```python
from build123d import *

# Parameters (mm, degrees)
F2_DEPTH = 25.4
F0_W     = 101.8392853439
F0_H     = 138.1853856146
F0_R     = 44.7370158625
F3_DEPTH = 25.4


with BuildPart() as f2:
    # F1 (on Right) → F2 (new body)
    with BuildSketch(Plane.YZ):
        with BuildLine():
            ThreePointArc((5.1872688346, 24.6414919816), (16.2456525152, 42.3484863922), (20.1080592166, 62.8645122051))
            ThreePointArc((20.1080592166, 62.8645122051), (-51.2286548469, 117.2754631001), (-84.8408640002, 34.0907424688))
            Line((-84.8408640002, 34.0907424688), (5.1872688346, 34.0907424688))
            Line((5.1872688346, 34.0907424688), (5.1872688346, 24.6414919816))
        make_face()
        with BuildLine():
            Line((5.1872688346, 34.0907424688), (-84.8408640002, 34.0907424688))
            ThreePointArc((-84.8408640002, 34.0907424688), (-42.2001575317, 6.7538301414), (5.1872688346, 24.6414919816))
            Line((5.1872688346, 24.6414919816), (5.1872688346, 34.0907424688))
        make_face()
        with BuildLine():
            ThreePointArc((5.1872688346, 24.6414919816), (-42.2001575317, 6.7538301414), (-84.8408640002, 34.0907424688))
            Line((-84.8408640002, 34.0907424688), (-98.5580086708, 34.0907424688))
            Line((-98.5580086708, 34.0907424688), (-98.5580086708, -30.617037788))
            Line((-98.5580086708, -30.617037788), (5.1872688346, -30.617037788))
            Line((5.1872688346, -30.617037788), (5.1872688346, 24.6414919816))
        make_face()
    extrude(amount=F2_DEPTH)

    # F0 (on Top) → F3 (join)
    with BuildSketch(Plane.XY):
        with Locations((-13.9607731253, -10.5434413999)):
            Rectangle(F0_W, F0_H)
        with Locations((-15.9663036466, 12.9214562476)):
            Circle(F0_R, mode=Mode.SUBTRACT)
    extrude(amount=F3_DEPTH)


solid = f2.part
```
Build history of the part. All positions in model axes, mm. A direction names the side the tool comes from. Give positions to 0.01 mm unless a question says otherwise; leave off trailing zeros. Loops run counter-clockwise (first coordinate to the right, second up) from the corner with the lowest first, then second, coordinate; pieces in that order, holes last.
Item 1: Slice it at A-A, the plane y = -23.5. List the corners of the cut face in (x, z), and give its area (3 significant figures).
Answers follow:
outline: (-64.88, 0) - (-41.94, 0) - (-41.94, 25.4) - (-64.88, 25.4) - close; (0, -30.62) - (25.4, -30.62) - (25.4, 0) - (36.96, 0) - (36.96, 25.4) - (25.4, 25.4) - (25.4, 117.81) - (0, 117.81) - close
area: 4,650 mm2
Item 2: Which spindle directions (+Z, -Z, +X, -X, +Y, -Y) get a long thin tool onto all of the face, cutting with end or side? Do faces 1 (the face through (31, -79.636, 13)), 2 (the face through (13, -98.558, 2)), 3 (the face through (-33, -79.636, 13)). Say none if no direction does.
Answers follow:
face 1: +Z, -Z, +X, -Y
face 2: +Z, -Z, +X, -X, -Y
face 3: +Z, -Z, -X, -Y
Item 3: Drill centre lines: line 1 (X direction, y = 5, z = 22); line 2 (X direction, y = -86, z = 24.5); line 3 (Y direction, x = 18.5, z = -2). Where is each one in solid material? Low to high.
Answers follow:
line 1: x = -64.88 to -60, 0 to 25.4, 28.06 to 36.96
line 2: x = 0 to 25.4
line 3: y = -98.56 to 5.19
Item 4: Slice it at D-D, the plane y = -2. List the corners of the cut face in (x, z).
Answers follow:
outline: (-64.88, 0) - (-58.14, 0) - (-58.14, 25.4) - (-64.88, 25.4) - close; (0, -30.62) - (25.4, -30.62) - (25.4, 107.65) - (0, 107.65) - close; (26.21, 0) - (36.96, 0) - (36.96, 25.4) - (26.21, 25.4) - close
Item 5: Pull direction X, two halves, no side cores. Call faces 4 (the face through (-64.88, -12, 13)), 5 (the face through (13, -47, -30.617)), 6 (the face through (13, 5.187, -3)): released by +X, released by -X, zero draft, split by the parting line, or undercut.
Answers follow:
face 4: released by -X
face 5: zero draft
face 6: undercut
Item 6: Slice it at C-C, the plane z = 3. List the corners of the cut face in (x, y).
Answers follow:
outline: (-64.88, -79.64) - (0, -79.64) - (0, -98.56) - (25.4, -98.56) - (25.4, -79.64) - (36.96, -79.64) - (36.96, 58.55) - (-64.88, 58.55) - close; hole (0, -28.87) - (0, 5.19) - (25.4, 5.19) - (25.4, -4.11) arc R44.74 ccw (long way) to start
Item 7: Flat gauge pins, fed straight in: pin 1 (1 mm diameter, centred on y = -62, z = 99.5, fed in from -X); pin 2 (7.5 mm diameter, centred on x = 11.5, z = -8, fed in from +Y); pin 3 (10 mm diameter, centred on x = -47, y = -15.5, fed in from +Z). Where does each tip first touch, or does it go through?
Answers follow:
pin 1: stops at x = 0
pin 2: stops at y = 5.19
pin 3: stops at z = 25.4
Item 8: Slice it at B-B, the plane x = 18. List the corners of the cut face in (y, z).
Answers follow:
outline: (-98.56, -30.62) - (5.19, -30.62) - (5.19, 24.64) arc R56.42 ccw (long way) to (-84.84, 34.09) - (-98.56, 34.09) - close; (42.04, 0) - (58.55, 0) - (58.55, 25.4) - (42.04, 25.4) - close
